Verification items for the finished model (mm, model axes). A direction names the side the tool comes from. Give positions to 0.01 mm unless a question says otherwise; leave off trailing zeros. Write each loop counter-clockwise with the first axis right and the second up, starting at its lowest first coordinate (ties: lowest second). Pieces come first, ordered by that corner, then holes.
from build123d import *

# Parameters (mm, degrees)
SKETCH1_W           = 43.18
SKETCH1_H           = 17.78
BOSS_EXTRUDE1_DEPTH = 12.7
CUT_EXTRUDE1_DEPTH  = 7.62
CUT_EXTRUDE2_DEPTH  = 49.393499563


with BuildPart() as part:
    # Sketch1 → Boss-Extrude1 (new body)
    with BuildSketch(Plane.XY):
        with Locations((21.59, 8.89)):
            Rectangle(SKETCH1_W, SKETCH1_H)
    extrude(amount=-BOSS_EXTRUDE1_DEPTH)

    # Sketch3 → Cut-Extrude1 (cut)
    with BuildSketch(Plane(origin=(0, 17.78, 0), x_dir=(1, 0, 0), z_dir=(0, 1, 0))):
        Polygon((43.18, 12.7), (36.83, 6.35), (43.18, 0), align=None)
    extrude(amount=-CUT_EXTRUDE1_DEPTH, mode=Mode.SUBTRACT)

    # Sketch4 → Cut-Extrude2 (cut, through all)
    with BuildSketch(Plane(origin=(0, 17.78, 0), x_dir=(1, 0, 0), z_dir=(0, 1, 0))):
        with BuildLine():
            Line((32.131, 3.556), (24.511, 3.556))
            ThreePointArc((24.511, 3.556), (21.717, 6.35), (24.511, 9.144))
            Line((24.511, 9.144), (32.131, 9.144))
            ThreePointArc((32.131, 9.144), (34.925, 6.35), (32.131, 3.556))
        make_face()
        with BuildLine():
            Line((13.843, 3.556), (6.223, 3.556))
            ThreePointArc((6.223, 3.556), (3.429, 6.35), (6.223, 9.144))
            Line((6.223, 9.144), (13.843, 9.144))
            ThreePointArc((13.843, 9.144), (16.637, 6.35), (13.843, 3.556))
        make_face()
    extrude(amount=-CUT_EXTRUDE2_DEPTH, mode=Mode.SUBTRACT)


solid = part.part
Item 1: Release check for a two-part mould opening along X. For faces 4 (the face through (39.96, 14.02, -3.22)), 5 (the face through (16.636, 9.014, -6.411)), 6 (the face through (41, 10.16, -6)), 7 (the face through (0, 9, -6)) record: released by +X, released by -X, zero draft, split by the parting line, or undercut.
Answer key:
face 4: released by +X
face 5: undercut
face 6: zero draft
face 7: released by -X
Item 2: Sectioned sample at B-B on y = 8.75. Record the cut outline in (x, z), then the cut area to 3 significant figures.
Answer key:
outline: (0, -12.7) - (43.18, -12.7) - (43.18, 0) - (0, 0) - close; hole (6.22, -9.14) - (13.84, -9.14) arc R2.79 ccw to (13.84, -3.56) - (6.22, -3.56) arc R2.79 ccw to start; hole (24.51, -9.14) - (32.13, -9.14) arc R2.79 ccw to (32.13, -3.56) - (24.51, -3.56) arc R2.79 ccw to start
area: 414 mm2
Item 3: Depth check by flat-ended pin: pin 1 (8.5 mm diameter, centred on x = 26.5, y = 5.5, fed in from +Z). Enter the tip coordinate at first touch or a pass-through.
Answer key:
pin 1: stops at z = 0
Item 4: Sectioned sample at D-D on y = 13.25. Record the cut outline in (x, z).
Answer key:
outline: (0, -12.7) - (43.18, -12.7) - (36.83, -6.35) - (43.18, 0) - (0, 0) - close; hole (6.22, -9.14) - (13.84, -9.14) arc R2.79 ccw to (13.84, -3.56) - (6.22, -3.56) arc R2.79 ccw to start; hole (24.51, -9.14) - (32.13, -9.14) arc R2.79 ccw to (32.13, -3.56) - (24.51, -3.56) arc R2.79 ccw to start
Item 5: Sectioned sample at A-A on x = 12. Record the cut outline in (y, z), then the cut area to 3 significant figures.
Answer key:
outline: (0, -12.7) - (17.78, -12.7) - (17.78, -9.14) - (0, -9.14) - close; (0, -3.56) - (17.78, -3.56) - (17.78, 0) - (0, 0) - close
area: 126 mm2
Item 6: Scan lines: line 1 along Z through (x, y) = (11, 7); line 2 along X through (y, z) = (10, -8.5); line 3 along X through (y, z) = (13, -4.5). Record each from-to range of solid material in increasing order.
Answer key:
line 1: z = -12.7 to -9.14, -3.56 to 0
line 2: x = 0 to 4.44, 15.63 to 22.73, 33.92 to 43.18
line 3: x = 0 to 4.13, 15.94 to 22.42, 34.22 to 38.68
Item 7: Sectioned sample at C-C on z = -10.75. Record the cut outline in (x, y).
Answer key:
outline: (0, 0) - (43.18, 0) - (43.18, 10.16) - (41.23, 10.16) - (41.23, 17.78) - (0, 17.78) - close
Item 8: Set-up check for faces 1 (the face through (3.43, 9.01, -6.29)), 2 (the face through (21, 9, -12.7)), 3 (the face through (40.05, 14.02, -9.57)): record each of +Z, -Z, +X, -X, +Y, -Y from which the full face is reachable in a straight line by a thin tool's end or side.
Answer key:
face 1: +Y, -Y
face 2: -Z, +X, -X, +Y, -Y
face 3: +X, +Y
